```python
from build123d import *

# Parameters (mm, degrees)
PAD_DEPTH              = 2.5
CYLINDER001_R          = 1.75
CYLINDER001_DEPTH      = 10
CYLINDER001_ROLL_ANGLE = 90
BOX_W                  = 6
BOX_H                  = 3
BOX_DEPTH              = 7.5
SKETCH003_R            = 2.75
PAD001_DEPTH           = 8
CHAMFER_SIZE           = 1.5
POCKET_DEPTH           = 218.644926
POLARPATTERN_COUNT     = 5


with BuildPart() as captive_nut:
    # Sketch002 → Pad (new body)
    with BuildSketch(Plane.XZ):
        Polygon((-2.875, 5), (2.875, 5), (2.875, -1.659882), (0, -3.319764), (-2.875, -1.659882), align=None)
    extrude(amount=PAD_DEPTH)


with BuildPart() as captive_nut_1:
    # Clone placement: moved
    add(captive_nut.part.moved(Location((0, -3.75, 2))))


with BuildPart() as captive_nut_screw_fusion:
    # Cylinder001 → Cylinder001 (new body)
    with BuildSketch(Plane.XY):
        Circle(CYLINDER001_R)
    extrude(amount=CYLINDER001_DEPTH)


with BuildPart() as captive_nut_screw_fusion_1:
    # Cylinder001 roll: moved
    add(captive_nut_screw_fusion.part.rotate(Axis((0, 0, 0), (1, 0, 0)), CYLINDER001_ROLL_ANGLE))


with BuildPart() as captive_nut_screw_fusion_2:
    # Cylinder001 placement: moved
    add(captive_nut_screw_fusion_1.part.moved(Location((0, 0, 2))))

    # Fusion: union captive-nut
    add(captive_nut_1.part)


with BuildPart() as captive_nut_screw_fusion_3:
    # Fusion placement: moved
    add(captive_nut_screw_fusion_2.part.moved(Location((0, 1.2, 0))))


with BuildPart() as shaft_recess_cube:
    # Box → Box (new body)
    with BuildSketch(Plane(origin=(-3, 1.625, -3), x_dir=(1, 0, 0), z_dir=(0, 0, 1))):
        with Locations((3, 1.5)):
            Rectangle(BOX_W, BOX_H)
    extrude(amount=BOX_DEPTH)


with BuildPart() as wheel_r:
    # Sketch → Revolution (revolve)
    with BuildSketch(Plane.XZ):
        Polygon((0, -2), (27.5, -2), (32.5, 3), (36.5, 3), (36.5, 2.12132), (34.37868, 0), (36.5, -2.12132), (36.5, -3), (34.5, -5), (0, -5), align=None)
    revolve(axis=Axis((0, 0, 0), (0, 0, 1)))

    # Sketch003 → Pad001 (new body)
    with BuildSketch(Plane(origin=(0, 0, -2), x_dir=(-1, 0, 0), z_dir=(0, 0, 1))):
        with BuildLine():
            ThreePointArc((-3.49106, 7.75), (0, -8.5), (3.49106, 7.75))
            Line((3.49106, 7.75), (-3.49106, 7.75))
        make_face()
        Circle(SKETCH003_R, mode=Mode.SUBTRACT)
    extrude(amount=PAD001_DEPTH)

    # Fusion001: union shaft-recess-cube
    add(shaft_recess_cube.part)

    # Cut: cut captive-nut-screw-fusion
    add(captive_nut_screw_fusion_3.part, mode=Mode.SUBTRACT)

    # Chamfer
    chamfer_edges = [wheel_r.edges().sort_by_distance(p)[0] for p in [
        (0, 8.5, -2),
    ]]
    chamfer(chamfer_edges, length=CHAMFER_SIZE)

    # Sketch004 → Pocket (cut, through all)
    with BuildSketch(Plane(origin=(0, 0, -5), x_dir=(1, 0, 0), z_dir=(0, 0, -1))):
        with BuildLine():
            ThreePointArc((-8.749102, 15.157148), (9.610963, 17.237864), (-4.842852, 28.749102))
            Line((-13.591954, 23.90625), (-4.842852, 28.749102))
            Line((-8.749102, 15.157148), (-13.591954, 23.90625))
        make_face()
    pocket = extrude(amount=-POCKET_DEPTH, mode=Mode.SUBTRACT)

    # PolarPattern: Pocket ×5 about axis
    polarpattern_axis = Axis((0, 0, -5), (0, 0, -1))
    for i in range(1, POLARPATTERN_COUNT):
        add(pocket.rotate(polarpattern_axis, i * 360 / POLARPATTERN_COUNT), mode=Mode.SUBTRACT)


solid = wheel_r.part
```
Build history of the part. All positions in model axes, mm. A direction names the side the tool comes from. Give positions to 0.01 mm unless a question says otherwise; leave off trailing zeros. One line per question, with ' | ' between items. Start each with the question number.
1) Cut at A-A (y = 0). Count the separate pieces of the cut face and the enclosed holes in it, plus the area to 3 significant figures.
2) 3-axis set-ups, long thin cutter, end or side, ignore diameter. For faces 1 (the flat face through (-11.137, -19.47, -3.521)), 2 (the flat face through (0, 1.625, 1)): which of +Z, -Z, +X, -X, +Y, -Y reach the whole face in a straight line?
3) Probe L1, parallel to Y at x = 4, z = 0.5; L2, parallel to X at y = 11.5, z = -3.5; L3, parallel to Z at x = -22.5, y = -25.5. List the from-to ranges inside material, lowest first.
4) Two-plate mould, pull along Z, no slides. Class faces 3 (the cylindrical face through (0.81, -6.38, 0.45)), 4 (the flat face through (0, -1, -2)), 5 (the flat face through (-2.435, 22.298, -3.521)): released by +Z, released by -Z, zero draft, split by the parting line, or undercut.
5) Pin check, flat tips, straight feed: pin 1 (3 mm diameter, centred on x = 1.5, z = 4, fed in from +Y); pin 2 (16 mm diameter, centred on x = 0, y = -20, fed in from -Z); pin 3 (8 mm diameter, centred on x = 8.5, y = 4.5, fed in from +Z); pin 4 (1.5 mm diameter, centred on x = 2, z = 3, fed in from -Y). Stop position of each tip, or through.
Return value:
1) separate pieces: 3 | enclosed holes: 0 | area: 267 mm^2
2) face 1: +Z, -Z | face 2: +Z
3) L1: -34.65 to -29.73, -7.5 to 7.5, 29.73 to 34.65 | L2: -34.11 to -20.59, -2.92 to 2.92, 24.98 to 34.11 | L3: -5 to 3
4) face 3: undercut | face 4: released by +Z | face 5: zero draft
5) pin 1: y = 36.5 | pin 2: through | pin 3: z = 6 | pin 4: y = -36.48
